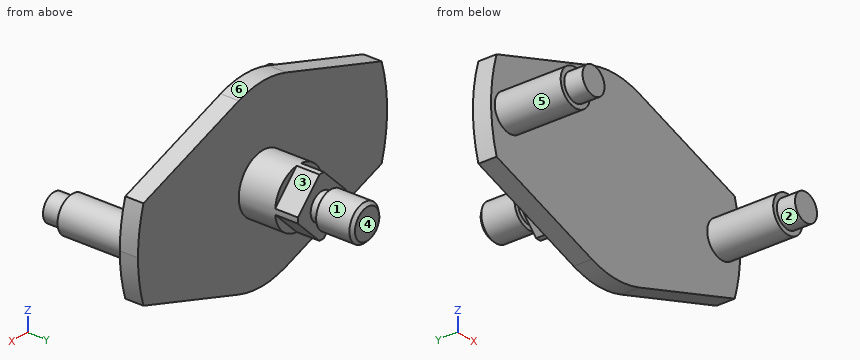
```python
from build123d import *

# Parameters (mm, degrees)
EXTRUDE_1_DEPTH      = 4
SKETCH_2_R           = 6.5
EXTRUDE_2_DEPTH      = 13
SKETCH_3_R           = 4
EXTRUDE_3_DEPTH      = 10
SKETCH_4_OUTSIDE_W   = 86.676
SKETCH_4_OUTSIDE_H   = 58.676
SKETCH_4_OUTSIDE_R   = 3
CUT_EXTRUDE_1_DEPTH  = 2
SKETCH_6_OUTSIDE_W   = 86.676
SKETCH_6_OUTSIDE_H   = 58.676
CUT_EXTRUDE_2_DEPTH  = 5
SKETCH_7_R           = 4
EXTRUDE_4_DEPTH      = 18.5
SKETCH_8_OUTSIDE_W   = 88.214
SKETCH_8_OUTSIDE_H   = 60.214
SKETCH_8_OUTSIDE_R   = 3
CUT_EXTRUDE_3_DEPTH  = 4
MIRROR_START         = -14.5
MIRROR_1_OUTLINE_R   = 4
MIRROR_1_DEPTH       = 14.5
MIRROR_START_2       = -18.5
MIRROR_1_2_OUTLINE_R = 3
MIRROR_1_2_DEPTH     = 4


# Read off the part's stored shape, not the designer's step: M8 机械螺纹 螺柱1, 镜向1
with BuildPart() as part:
    # 草图1 → 凸台-拉伸1 (new body)
    with BuildSketch(Plane(origin=(0, 0, 0), x_dir=(1, 0, 0), z_dir=(0, 1, 0))):
        with BuildLine():
            Line((-6.487344821, 18.918624611), (-32.496153619, 10))
            ThreePointArc((-32.496153619, 10), (-34, 0), (-32.496153619, -10))
            Line((-32.496153619, -10), (-6.487344821, -18.918624611))
            ThreePointArc((-6.487344821, -18.918624611), (0, -20), (6.487344821, -18.918624611))
            Line((6.487344821, -18.918624611), (32.496153619, -10))
            ThreePointArc((32.496153619, -10), (33.621936463, -5.056222749), (34, 0))
            ThreePointArc((34, 0), (33.621936463, 5.056222749), (32.496153619, 10))
            Line((32.496153619, 10), (6.487344821, 18.918624611))
            ThreePointArc((6.487344821, 18.918624611), (0, 20), (-6.487344821, 18.918624611))
        make_face()
    extrude(amount=EXTRUDE_1_DEPTH)

    # 草图2 → 凸台-拉伸2 (add)
    with BuildSketch(Plane(origin=(0, 4, 0), x_dir=(1, 0, 0), z_dir=(0, 1, 0))):
        with Locations(Location((0, 0, 0), (0, 0, 90))):
            Circle(SKETCH_2_R)
    extrude(amount=EXTRUDE_2_DEPTH)

    # 草图3 → 凸台-拉伸3 (add)
    with BuildSketch(Plane(origin=(0, 17, 0), x_dir=(1, 0, 0), z_dir=(0, 1, 0))):
        with Locations(Location((0, 0, 0), (0, 0, 270))):
            Circle(SKETCH_3_R)
    extrude(amount=EXTRUDE_3_DEPTH)

    # 草图4 outside → 切除-拉伸1 (cut)
    with BuildSketch(Plane(origin=(0, 17, 0), x_dir=(1, 0, 0), z_dir=(0, 1, 0))):
        Rectangle(SKETCH_4_OUTSIDE_W, SKETCH_4_OUTSIDE_H)
        with Locations(Location((0, 0, 0), (0, 0, 270))):
            Circle(SKETCH_4_OUTSIDE_R, mode=Mode.SUBTRACT)
    extrude(amount=CUT_EXTRUDE_1_DEPTH, mode=Mode.SUBTRACT)

    # M8 机械螺纹 螺柱1 outline → M8 机械螺纹 螺柱1 (revolve, cut)
    with BuildSketch(Plane.XY):
        Polygon((4, 27), (3.3235, 27), (4, 26.3235), align=None)
    revolve(axis=Axis((0, 0, 0), (0, 1, 0)), mode=Mode.SUBTRACT)

    # 草图6 outside → 切除-拉伸2 (cut)
    with BuildSketch(Plane(origin=(0, 17, 0), x_dir=(1, 0, 0), z_dir=(0, 1, 0))):
        Rectangle(SKETCH_6_OUTSIDE_W, SKETCH_6_OUTSIDE_H)
        Polygon((0, -7.071067812), (7.071067812, 0), (0, 7.071067812), (-7.071067812, 0), align=None, mode=Mode.SUBTRACT)
    extrude(amount=-CUT_EXTRUDE_2_DEPTH, mode=Mode.SUBTRACT)

    # 草图7 → 凸台-拉伸4 (add)
    with BuildSketch(Plane.XZ):
        with Locations(Location((29, 0, 0), (0, 0, 90))):
            Circle(SKETCH_7_R)
    extrude(amount=EXTRUDE_4_DEPTH)

    # 草图8 outside → 切除-拉伸3 (cut)
    with BuildSketch(Plane.XZ.offset(18.5)):
        Rectangle(SKETCH_8_OUTSIDE_W, SKETCH_8_OUTSIDE_H)
        with Locations(Location((29, 0, 0), (0, 0, 270))):
            Circle(SKETCH_8_OUTSIDE_R, mode=Mode.SUBTRACT)
    extrude(amount=-CUT_EXTRUDE_3_DEPTH, mode=Mode.SUBTRACT)

    # 镜向1 outline → 镜向1 (add)
    with BuildSketch(Plane(origin=(0, 0, 0), x_dir=(1, 0, 0), z_dir=(0, 1, 0)).offset(MIRROR_START)):
        with Locations((-29, 0)):
            Circle(MIRROR_1_OUTLINE_R)
    extrude(amount=MIRROR_1_DEPTH)

    # Mirror 1 2 outline → Mirror 1 2 (add)
    with BuildSketch(Plane(origin=(0, 0, 0), x_dir=(1, 0, 0), z_dir=(0, 1, 0)).offset(MIRROR_START_2)):
        with Locations((-29, 0)):
            Circle(MIRROR_1_2_OUTLINE_R)
    extrude(amount=MIRROR_1_2_DEPTH)


solid = part.part
```
The model under review builds one solid part; all positions refer to its coordinate system, in mm. Face numbers are marked on the shaded views. A direction names the side the tool comes from. Round coordinates to 2 decimals unless told otherwise and drop trailing zeros. Order: outer loops, then holes, each group sorted by start corner. A loop starts at its lowest first (then second) coordinate and runs counter-clockwise, first axis right, second up.
Item 1: Draft analysis for pull direction X (two halves, no side actions). For the marked faces 4, 5 and 6, state which applies: released by +X, released by -X, zero draft, split by the parting line, or undercut.
Working result:
face 4: zero draft
face 5: undercut
face 6: split by the parting line
Item 2: To check wall thickness, follow probe 1 along Y at (x, z) = (-8, 1); probe 2 along Y at (x, z) = (2.5, -5); probe 3 along X at (y, z) = (16.5, -0.5). State the ranges of each line that lie inside material, in increasing order.
Working result:
probe 1: y = 0 to 4
probe 2: y = 0 to 12
probe 3: x = -6.48 to 6.48
Item 3: For pin 1 (20 mm diameter, centred on x = 6.5, z = 5, fed in from -Y); pin 2 (12 mm diameter, centred on x = 27, y = -10.5, fed in from +Z); pin 3 (2 mm diameter, centred on x = 25.5, z = -11, fed in from +Y), all flat-tipped, find the tip position at first contact; note any pin that passes through.
Working result:
pin 1: stops at y = 0
pin 2: stops at z = 4
pin 3: stops at y = 4
Item 4: Add section D-D, the plane z = -13.5. State the section outline as (x, y) points, and give its area (3 significant figures).
Working result:
outline: (-22.29, 0) - (22.29, 0) - (22.29, 4) - (-22.29, 4) - close
area: 178 mm2
Item 5: Machinability: for the marked faces 1, 2 and 3, which of the approach directions +Z, -Z, +X, -X, +Y, -Y give a long, thin tool a straight path to every point of the face, cutting with its end or side? Answer none if there is none.
Working result:
face 1: +Y
face 2: -Y
face 3: +Z, +X, +Y
Item 6: Add section C-C, the plane y = 8. State the section outline as (x, z) points.
Working result:
outline: circle Ø13 at (0, 0)
Item 7: Add section A-A, the plane y = -11. State the section outline as (x, z) points, and give its area (3 significant figures).
Working result:
outline: circle Ø8 at (-29, 0); circle Ø8 at (29, 0)
area: 101 mm2
Item 8: Add section B-B, the plane x = -29. State the section outline as (y, z) points.
Working result:
outline: (-18.5, -3) - (-14.5, -3) - (-14.5, -4) - (0, -4) - (0, -11.2) - (4, -11.2) - (4, 11.2) - (0, 11.2) - (0, 4) - (-14.5, 4) - (-14.5, 3) - (-18.5, 3) - close
